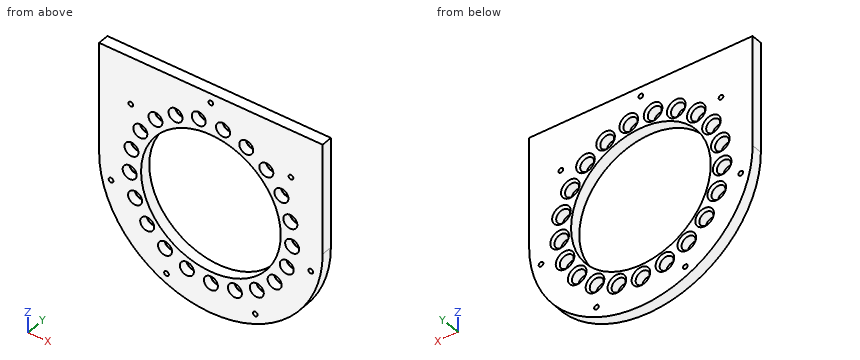
from build123d import *

# Parameters (mm, degrees)
SKETCH17_W          = 96
SKETCH17_H          = 48
BOSS_EXTRUDE1_DEPTH = 4.7625
SKETCH2_R           = 48
SKETCH2_R_2         = 3
SKETCH2_R_3         = 1
SKETCH2_R_4         = 30
BOSS_EXTRUDE2_DEPTH = 4.7625
SKETCH2_11_R        = 3
SKETCH2_11_R_2      = 1
SKETCH2_11_R_3      = 30
CUT_EXTRUDE1_DEPTH  = 4.7625
CHAMFER1_SIZE       = 1


with BuildPart() as part:
    # Sketch17 → Boss-Extrude1 (new body)
    with BuildSketch(Plane(origin=(0, 0, 0), x_dir=(1, 0, 0), z_dir=(0, 1, 0))):
        with Locations((0, -24)):
            Rectangle(SKETCH17_W, SKETCH17_H)
    extrude(amount=BOSS_EXTRUDE1_DEPTH)

    # Sketch2 → Boss-Extrude2 (add)
    with BuildSketch(Plane(origin=(0, 0, 0), x_dir=(1, 0, 0), z_dir=(0, 1, 0))):
        Circle(SKETCH2_R)
        with Locations(Location((0, 35, 0), (0, 0, 90))):
            Circle(SKETCH2_R_2, mode=Mode.SUBTRACT)
        with Locations(Location((10.316431104, 33.445048203, 0), (0, 0, 90))):
            Circle(SKETCH2_R_2, mode=Mode.SUBTRACT)
        with Locations(Location((19.716202032, 28.918357101, 0), (0, 0, 90))):
            Circle(SKETCH2_R_2, mode=Mode.SUBTRACT)
        with Locations(Location((27.364101886, 21.822143065, 0), (0, 0, 90))):
            Circle(SKETCH2_R_2, mode=Mode.SUBTRACT)
        with Locations(Location((32.580581203, 12.786935853, 0), (0, 0, 90))):
            Circle(SKETCH2_R_2, mode=Mode.SUBTRACT)
        with Locations((34.902132901, 2.615553276)):
            Circle(SKETCH2_R_2, mode=Mode.SUBTRACT)
        with Locations((34.122476926, -7.788232688)):
            Circle(SKETCH2_R_2, mode=Mode.SUBTRACT)
        with Locations((30.310889132, -17.5)):
            Circle(SKETCH2_R_2, mode=Mode.SUBTRACT)
        with Locations((23.806045822, -25.656815514)):
            Circle(SKETCH2_R_2, mode=Mode.SUBTRACT)
        with Locations((15.185930869, -31.533910377)):
            Circle(SKETCH2_R_2, mode=Mode.SUBTRACT)
        with Locations((5.216479316, -34.609078918)):
            Circle(SKETCH2_R_2, mode=Mode.SUBTRACT)
        with Locations((-5.216479316, -34.609078918)):
            Circle(SKETCH2_R_2, mode=Mode.SUBTRACT)
        with Locations((-15.185930869, -31.533910377)):
            Circle(SKETCH2_R_2, mode=Mode.SUBTRACT)
        with Locations((-23.806045822, -25.656815514)):
            Circle(SKETCH2_R_2, mode=Mode.SUBTRACT)
        with Locations((-30.310889132, -17.5)):
            Circle(SKETCH2_R_2, mode=Mode.SUBTRACT)
        with Locations((-34.122476926, -7.788232688)):
            Circle(SKETCH2_R_2, mode=Mode.SUBTRACT)
        with Locations((0, -44)):
            Circle(SKETCH2_R_3, mode=Mode.SUBTRACT)
        with Locations((-34.400585229, -27.433551282)):
            Circle(SKETCH2_R_3, mode=Mode.SUBTRACT)
        with Locations(Location((-42.896828136, 9.790921094, 0), (0, 0, 90))):
            Circle(SKETCH2_R_3, mode=Mode.SUBTRACT)
        with Locations(Location((-19.090884521, 39.642630188, 0), (0, 0, 90))):
            Circle(SKETCH2_R_3, mode=Mode.SUBTRACT)
        with Locations(Location((19.090884521, 39.642630188, 0), (0, 0, 90))):
            Circle(SKETCH2_R_3, mode=Mode.SUBTRACT)
        with Locations(Location((42.896828136, 9.790921094, 0), (0, 0, 90))):
            Circle(SKETCH2_R_3, mode=Mode.SUBTRACT)
        with Locations((34.400585229, -27.433551282)):
            Circle(SKETCH2_R_3, mode=Mode.SUBTRACT)
        with Locations((-34.902132901, 2.615553276)):
            Circle(SKETCH2_R_2, mode=Mode.SUBTRACT)
        with Locations(Location((-32.580581203, 12.786935853, 0), (0, 0, 90))):
            Circle(SKETCH2_R_2, mode=Mode.SUBTRACT)
        with Locations(Location((-27.364101886, 21.822143065, 0), (0, 0, 90))):
            Circle(SKETCH2_R_2, mode=Mode.SUBTRACT)
        with Locations(Location((-19.716202032, 28.918357101, 0), (0, 0, 90))):
            Circle(SKETCH2_R_2, mode=Mode.SUBTRACT)
        with Locations(Location((-10.316431104, 33.445048203, 0), (0, 0, 90))):
            Circle(SKETCH2_R_2, mode=Mode.SUBTRACT)
        Circle(SKETCH2_R_4, mode=Mode.SUBTRACT)
    extrude(amount=BOSS_EXTRUDE2_DEPTH)

    # Sketch2_11 → Cut-Extrude1 (cut)
    with BuildSketch(Plane(origin=(0, 0, 0), x_dir=(1, 0, 0), z_dir=(0, 1, 0))):
        with Locations(Location((34.902132901, 2.615553276, 0), (0, 0, 90))):
            Circle(SKETCH2_11_R)
        with Locations(Location((34.122476926, -7.788232688, 0), (0, 0, 90))):
            Circle(SKETCH2_11_R)
        with Locations(Location((30.310889132, -17.5, 0), (0, 0, 90))):
            Circle(SKETCH2_11_R)
        with Locations(Location((23.806045822, -25.656815514, 0), (0, 0, 90))):
            Circle(SKETCH2_11_R)
        with Locations(Location((15.185930869, -31.533910377, 0), (0, 0, 90))):
            Circle(SKETCH2_11_R)
        with Locations(Location((5.216479316, -34.609078918, 0), (0, 0, 90))):
            Circle(SKETCH2_11_R)
        with Locations(Location((-5.216479316, -34.609078918, 0), (0, 0, 90))):
            Circle(SKETCH2_11_R)
        with Locations(Location((-15.185930869, -31.533910377, 0), (0, 0, 90))):
            Circle(SKETCH2_11_R)
        with Locations(Location((-23.806045822, -25.656815514, 0), (0, 0, 90))):
            Circle(SKETCH2_11_R)
        with Locations(Location((-30.310889132, -17.5, 0), (0, 0, 90))):
            Circle(SKETCH2_11_R)
        with Locations(Location((-34.122476926, -7.788232688, 0), (0, 0, 90))):
            Circle(SKETCH2_11_R)
        with Locations(Location((0, -44, 0), (0, 0, 90))):
            Circle(SKETCH2_11_R_2)
        with Locations(Location((-34.400585229, -27.433551282, 0), (0, 0, 90))):
            Circle(SKETCH2_11_R_2)
        with Locations(Location((34.400585229, -27.433551282, 0), (0, 0, 90))):
            Circle(SKETCH2_11_R_2)
        with Locations(Location((-34.902132901, 2.615553276, 0), (0, 0, 90))):
            Circle(SKETCH2_11_R)
        with Locations(Location((0, 0, 0), (0, 0, 90))):
            Circle(SKETCH2_11_R_3)
    extrude(amount=CUT_EXTRUDE1_DEPTH, mode=Mode.SUBTRACT)

    # Chamfer1
    chamfer1_edges = [part.edges().sort_by_distance(p)[0] for p in [
        (-30.310889132, 4.7625, 20.5),
        (-23.806045822, 4.7625, 28.656815514),
        (-15.185930869, 4.7625, 34.533910377),
        (-5.216479316, 4.7625, 37.609078918),
        (5.216479316, 4.7625, 37.609078918),
        (15.185930869, 4.7625, 34.533910377),
        (23.806045822, 4.7625, 28.656815514),
        (30.310889132, 4.7625, 20.5),
        (34.122476926, 4.7625, 10.788232688),
        (-34.122476926, 4.7625, 10.788232688),
        (36.371446028, 4.7625, -5.231106551),
        (-33.432819775, 4.7625, -5.231106551),
        (0, 4.7625, -32),
        (10.316431104, 4.7625, -30.445048203),
        (19.716202032, 4.7625, -25.918357101),
        (27.364101886, 4.7625, -18.822143065),
        (32.580581203, 4.7625, -9.786935853),
        (-32.580581203, 4.7625, -9.786935853),
        (-27.364101886, 4.7625, -18.822143065),
        (-19.716202032, 4.7625, -25.918357101),
        (-10.316431104, 4.7625, -30.445048203),
    ]]
    chamfer(chamfer1_edges, length=CHAMFER1_SIZE)


solid = part.part
The listing builds one solid part. Answer for the finished solid, in the listing's coordinates (mm). Round coordinates to 2 decimals unless told otherwise and drop trailing zeros. Write each loop counter-clockwise with the first axis right and the second up, starting at its lowest first coordinate (ties: lowest second). Pieces come first, ordered by that corner, then holes. Notation, with made-up numbers: (-37, 1.25) - (10, 1.25) arc R33 ccw to (10, 35.25) - close; hole circle Ø1 at (26.5, -37). An arc over 180 degrees is marked (long way). Use a Markdown table: item, result. Add a question column.
1. Flat-ended cylindrical pins translate along their axes: P1, Ø5.5, axis at x = -32.58, z = -12.79, coming from the -Y side; P2, Ø2, axis at x = -34.5, y = 1, coming from the -Z side. Find the tip coordinate at first contact, or state that the pin passes through.
2. Consider line 1 (X direction, y = 1, z = 17.5); line 2 (Z direction, x = -5.5, y = 3.15); line 3 (X direction, y = 2.15, z = -1.5). Determine where each line is inside the solid, lowest interval first.
3. The part is cut by section A-A (z = 17.5). Write down the section's boundary in (x, y), and give its area (3 significant figures).
4. The part is cut by section B-B (y = 1.9). Give the number of separate pieces and of enclosed holes in the cut face, and give its area (3 significant figures).
Reported:
| question | item | result |
|---|---|---|
| 1 | P1 | through |
| 1 | P2 | z = -34.38 |
| 2 | line 1 | -48 to -33.31, -27.31 to -24.37, 24.37 to 27.31, 33.31 to 48 |
| 2 | line 2 | -47.68 to -29.49, 29.49 to 31.62, 37.6 to 48 |
| 2 | line 3 | -47.98 to -37.69, -32.12 to -29.96, 29.96 to 32.12, 37.69 to 47.98 |
| 3 | outline | (-48, 0) - (-33.31, 0) - (-33.31, 3.76) - (-34.31, 4.76) - (-48, 4.76) - close; (-27.31, 0) - (-24.37, 0) - (-24.37, 4.76) - (-26.31, 4.76) - (-27.31, 3.76) - close; (24.37, 0) - (27.31, 0) - (27.31, 3.76) - (26.31, 4.76) - (24.37, 4.76) - close; (33.31, 0) - (48, 0) - (48, 4.76) - (34.31, 4.76) - (33.31, 3.76) - close |
| 3 | area | 166 mm^2 |
| 4 | separate pieces | 1 |
| 4 | enclosed holes | 29 |
| 4 | area | 4,780 mm^2 |
